Could you check a few things on this model? Use its own coordinates, in mm. A direction names the side the tool comes from. Coordinates: 2 decimals unless noted, no trailing zeros. Loops run counter-clockwise (first coordinate to the right, second up) from the corner with the lowest first, then second, coordinate; pieces in that order, holes last.
1) Thinking about a two-plate mould opening in Z: for faces 1 (the face through (-1, 0, 0)), 2 (the face through (-46.859, 1.61, -20.297)), 3 (the face through (-40.467, 1.565, -0.267)), which applies, released by +Z, released by -Z, zero draft, split by the parting line, or undercut?
2) Imagine slicing it at B-B on z = 16. Please give me the cut outline in (x, y) (3 decimals), plus the area to 3 significant figures.
3) Imagine slicing it at A-A on x = 34. Please give me the cut outline in (y, z) (3 decimals).
4) Imagine slicing it at D-D on x = 20.5. Please give me the cut outline in (y, z) (3 decimals).
5) Will this pin go through, and if not, where does the flat tip stop? P1, Ø2.5, axis at x = 42.5, z = 16, coming from the -Y side.
6) If I drill on line 1 along Z through (x, y) = (42.5, 2.25); line 2 along X through (y, z) = (1.2, -16); line 3 along X through (y, z) = (1.75, -1), over which ranges is the centre line in solid material (lowest first)?
7) For faces 4 (the face through (-1, 2, 21.5)), 5 (the face through (-1.65, 1.57, -15.95)), which set-ups out of +Z, -Z, +X, -X, +Y, -Y let a thin tool reach every point of the face, with its end or its side?
8) Imagine slicing it at C-C on x = -42.5. Please give me the cut outline in (y, z) (3 decimals), plus the area to 3 significant figures.
```python
from build123d import *

# Parameters (mm, degrees)
SKETCH1_W           = 96
SKETCH1_H           = 43
SKETCH1_R           = 8.05
SKETCH1_R_2         = 2.05
BOSS_EXTRUDE1_DEPTH = 3.175
FILLET1_R           = 4


with BuildPart() as part:
    # Sketch1 → Boss-Extrude1 (new body)
    with BuildSketch(Plane(origin=(0, 0, 0), x_dir=(1, 0, 0), z_dir=(0, 1, 0))):
        Rectangle(SKETCH1_W, SKETCH1_H)
        with Locations(Location((17.9, 0, 0), (0, 0, 270))):
            Circle(SKETCH1_R, mode=Mode.SUBTRACT)
        with Locations(Location((-17.9, 0, 0), (0, 0, 270))):
            Circle(SKETCH1_R_2, mode=Mode.SUBTRACT)
        with Locations(Location((-42.5, 16, 0), (0, 0, 270))):
            Circle(SKETCH1_R_2, mode=Mode.SUBTRACT)
        with Locations(Location((-42.5, 8, 0), (0, 0, 270))):
            Circle(SKETCH1_R_2, mode=Mode.SUBTRACT)
        with Locations(Location((-42.5, 0, 0), (0, 0, 270))):
            Circle(SKETCH1_R_2, mode=Mode.SUBTRACT)
        with Locations(Location((-42.5, -8, 0), (0, 0, 270))):
            Circle(SKETCH1_R_2, mode=Mode.SUBTRACT)
        with Locations(Location((-42.5, -16, 0), (0, 0, 270))):
            Circle(SKETCH1_R_2, mode=Mode.SUBTRACT)
        with Locations(Location((42.5, 16, 0), (0, 0, 90))):
            Circle(SKETCH1_R_2, mode=Mode.SUBTRACT)
        with Locations(Location((42.5, 8, 0), (0, 0, 90))):
            Circle(SKETCH1_R_2, mode=Mode.SUBTRACT)
        with Locations(Location((42.5, 0, 0), (0, 0, 90))):
            Circle(SKETCH1_R_2, mode=Mode.SUBTRACT)
        with Locations(Location((42.5, -8, 0), (0, 0, 90))):
            Circle(SKETCH1_R_2, mode=Mode.SUBTRACT)
        with Locations(Location((42.5, -16, 0), (0, 0, 90))):
            Circle(SKETCH1_R_2, mode=Mode.SUBTRACT)
        with BuildLine():
            Line((0.4, 18.05), (3.4, 18.05))
            ThreePointArc((3.4, 18.05), (5.45, 16), (3.4, 13.95))
            Line((3.4, 13.95), (0.4, 13.95))
            ThreePointArc((0.4, 13.95), (-1.65, 16), (0.4, 18.05))
        make_face(mode=Mode.SUBTRACT)
        with BuildLine():
            Line((0.4, -13.95), (3.4, -13.95))
            ThreePointArc((3.4, -13.95), (5.45, -16), (3.4, -18.05))
            Line((3.4, -18.05), (0.4, -18.05))
            ThreePointArc((0.4, -18.05), (-1.65, -16), (0.4, -13.95))
        make_face(mode=Mode.SUBTRACT)
        with BuildLine():
            Line((35.4, -18.05), (32.4, -18.05))
            ThreePointArc((32.4, -18.05), (30.35, -16), (32.4, -13.95))
            Line((32.4, -13.95), (35.4, -13.95))
            ThreePointArc((35.4, -13.95), (37.45, -16), (35.4, -18.05))
        make_face(mode=Mode.SUBTRACT)
        with BuildLine():
            Line((35.4, 13.95), (32.4, 13.95))
            ThreePointArc((32.4, 13.95), (30.35, 16), (32.4, 18.05))
            Line((32.4, 18.05), (35.4, 18.05))
            ThreePointArc((35.4, 18.05), (37.45, 16), (35.4, 13.95))
        make_face(mode=Mode.SUBTRACT)
    extrude(amount=BOSS_EXTRUDE1_DEPTH)

    # Fillet1
    fillet1_edges = [part.edges().sort_by_distance(p)[0] for p in [
        (-48, 1.5875, -21.5),
        (48, 1.5875, -21.5),
        (48, 1.5875, 21.5),
        (-48, 1.5875, 21.5),
    ]]
    fillet(fillet1_edges, radius=FILLET1_R)


solid = part.part
```
Filled in:
1. face 1: zero draft
1. face 2: released by -Z
1. face 3: undercut
2. outline: (-48, 0) - (-44.55, 0) - (-44.55, 3.175) - (-48, 3.175) - close; (-40.45, 0) - (-1.65, 0) - (-1.65, 3.175) - (-40.45, 3.175) - close; (5.45, 0) - (30.35, 0) - (30.35, 3.175) - (5.45, 3.175) - close; (37.45, 0) - (40.45, 0) - (40.45, 3.175) - (37.45, 3.175) - close; (44.55, 0) - (48, 0) - (48, 3.175) - (44.55, 3.175) - close
2. area: 234 mm2
3. outline: (0, -21.5) - (3.175, -21.5) - (3.175, -18.05) - (0, -18.05) - close; (0, -13.95) - (3.175, -13.95) - (3.175, 13.95) - (0, 13.95) - close; (0, 18.05) - (3.175, 18.05) - (3.175, 21.5) - (0, 21.5) - close
4. outline: (0, -21.5) - (3.175, -21.5) - (3.175, -7.619) - (0, -7.619) - close; (0, 7.619) - (3.175, 7.619) - (3.175, 21.5) - (0, 21.5) - close
5. P1: passes through
6. line 1: z = -21.5 to -18.05, -13.95 to -10.05, -5.95 to -2.05, 2.05 to 5.95, 10.05 to 13.95, 18.05 to 21.5
6. line 2: x = -48 to -44.55, -40.45 to -1.65, 5.45 to 30.35, 37.45 to 40.45, 44.55 to 48
6. line 3: x = -48 to -44.29, -40.71 to -19.69, -16.11 to 9.91, 25.89 to 40.71, 44.29 to 48
7. face 4: +Z, +X, -X, +Y, -Y
7. face 5: +Y, -Y
8. outline: (0, -21.5) - (3.175, -21.5) - (3.175, -18.05) - (0, -18.05) - close; (0, -13.95) - (3.175, -13.95) - (3.175, -10.05) - (0, -10.05) - close; (0, -5.95) - (3.175, -5.95) - (3.175, -2.05) - (0, -2.05) - close; (0, 2.05) - (3.175, 2.05) - (3.175, 5.95) - (0, 5.95) - close; (0, 10.05) - (3.175, 10.05) - (3.175, 13.95) - (0, 13.95) - close; (0, 18.05) - (3.175, 18.05) - (3.175, 21.5) - (0, 21.5) - close
8. area: 71.4 mm2
